```python
from build123d import *

# Parameters (mm, degrees)
SKETCH1_R           = 18.5
BOSS_EXTRUDE1_DEPTH = 390
SKETCH2_R           = 3.175
BOSS_EXTRUDE2_DEPTH = 410


with BuildPart() as part:
    # Sketch1 → Boss-Extrude1 (new, symmetric)
    with BuildSketch(Plane.XY):
        Circle(SKETCH1_R)
    extrude(amount=BOSS_EXTRUDE1_DEPTH, both=True)

    # Sketch2 → Boss-Extrude2 (add, symmetric)
    with BuildSketch(Plane.XY):
        with Locations(Location((0, 0, 0), (0, 0, 180))):
            Circle(SKETCH2_R)
    extrude(amount=BOSS_EXTRUDE2_DEPTH, both=True)


solid = part.part
```
For this review, take the finished solid that the model builds, in its own axes (mm). Coordinates: 2 decimals unless noted, no trailing zeros. Order: outer loops, then holes, each group sorted by start corner. A loop starts at its lowest first (then second) coordinate and runs counter-clockwise, first axis right, second up. Notation, with made-up numbers: (60, -5) -> (96, -5) arc R24 ccw to (96, 19) -> close; hole circle Ø6 at (79, 5). An arc over 180 degrees is marked (long way). Answer as CSV lines item,"result".
Q1. We need section B-B (x = 11.5). State the section outline as (y, z) points.
Model answer:
outline,"(-14.49, -390) -> (14.49, -390) -> (14.49, 390) -> (-14.49, 390) -> close"
Q2. Clearance check with flat-ended pins moving along their axes: pin 1 Ø12 at (y, z) = (-7, 149.5) entering from +X; pin 2 Ø12 at (x, z) = (1, 6.5) entering from +Y; pin 3 Ø6 at (y, z) = (7, 48) entering from -X; pin 4 Ø12 at (x, y) = (-6.5, 3.5) entering from +Z. State where each tip first meets the part, or that it passes through.
Model answer:
pin 1,"stops at x = 18.47"
pin 2,"stops at y = 18.5"
pin 3,"stops at x = -18.06"
pin 4,"stops at z = 410"
Q3. Wall thickness on line 1 along Z through (x, y) = (13, -12); line 2 along Y through (x, z) = (1, -27.5); line 3 along Y through (x, z) = (-1.5, -137): over which ranges is each line inside the solid? List them lowest first. Write a range as [from, to].
Model answer:
line 1,"z = [-390, 390]"
line 2,"y = [-18.47, 18.47]"
line 3,"y = [-18.44, 18.44]"
Q4. We need section A-A (z = 198). State the section outline as (x, y) points.
Model answer:
outline,"circle Ø37 at (0, 0)"
